For this review, take the finished solid that the model builds, in its own axes (mm). Coordinates: 2 decimals unless noted, no trailing zeros. Write each loop counter-clockwise with the first axis right and the second up, starting at its lowest first coordinate (ties: lowest second). Pieces come first, ordered by that corner, then holes. Notation, with made-up numbers: M 17,52 L 29,52 A15 ccw 29,59 Z; hole C 28.5,17.5 d3. An arc over 180 degrees is marked long. One line per question, with ' | ' between items.
from build123d import *

# Parameters (mm, degrees)
RESSALTO_EXTRUS_O1_DEPTH = 6
FILETE1_R                = 80
CORTE_EXTRUS_O1_DEPTH    = 496.818515185
FILETE2_R                = 80
CORTE_EXTRUS_O2_DEPTH    = 496.818515327
CORTE_EXTRUS_O3_DEPTH    = 6
ESBO_O7_W                = 100
ESBO_O7_H                = 10
RESSALTO_EXTRUS_O4_DEPTH = 6


with BuildPart() as part:
    # Esboço1 → Ressalto-extrusão1 (new body)
    with BuildSketch(Plane.XY):
        Polygon((-150, 70), (0, 70), (0, 0), (180, 0), (180, 70), (330, 70), (330, 370), (-150, 370), align=None)
    extrude(amount=RESSALTO_EXTRUS_O1_DEPTH)

    # Filete1
    filete1_edges = [part.edges().sort_by_distance(p)[0] for p in [
        (-150, 370, 3),
        (330, 370, 3),
    ]]
    fillet(filete1_edges, radius=FILETE1_R)

    # Esboço4 → Corte-extrusão1 (cut, through all)
    with BuildSketch(Plane.XY.offset(6)):
        with BuildLine():
            Line((-150, 70), (0, 70))
            ThreePointArc((0, 70), (-36.716416622, 160.567770202), (-126.135181443, 200))
            Line((-126.135181443, 200), (-150, 200))
            Line((-150, 200), (-150, 70))
        make_face()
        with BuildLine():
            Line((330, 200), (306.135181443, 200))
            ThreePointArc((306.135181443, 200), (216.716416622, 160.567770202), (180, 70))
            Line((180, 70), (330, 70))
            Line((330, 70), (330, 200))
        make_face()
    extrude(amount=-CORTE_EXTRUS_O1_DEPTH, mode=Mode.SUBTRACT)

    # Filete2
    filete2_edges = [part.edges().sort_by_distance(p)[0] for p in [
        (330, 200, 3),
        (-150, 200, 3),
    ]]
    fillet(filete2_edges, radius=FILETE2_R)

    # Esboço5 → Corte-extrusão2 (cut, through all)
    with BuildSketch(Plane.XY.offset(6)):
        with BuildLine():
            Line((254.973969337, 280), (-76.120192614, 280))
            ThreePointArc((-76.120192614, 280), (-81.120192614, 275), (-76.120192614, 270))
            Line((-76.120192614, 270), (254.973969337, 270))
            ThreePointArc((254.973969337, 270), (259.973969337, 275), (254.973969337, 280))
        make_face()
    extrude(amount=-CORTE_EXTRUS_O2_DEPTH, mode=Mode.SUBTRACT)

    # Esboço6 → Corte-extrusão3 (cut)
    with BuildSketch(Plane.XY.offset(6)):
        with BuildLine():
            Line((50, 70), (130, 70.020316047))
            ThreePointArc((130, 70.020316047), (144.44257782, 140.677589128), (185.453428357, 200))
            Line((185.453428357, 200), (-5.474624038, 200))
            ThreePointArc((-5.474624038, 200), (35.551661067, 140.670775275), (50, 70))
        make_face()
    extrude(amount=-CORTE_EXTRUS_O3_DEPTH, mode=Mode.SUBTRACT)

    # Esboço7 → Ressalto-extrusão4 (add)
    with BuildSketch(Plane.XY.offset(6)):
        with Locations((89.426888362, 275)):
            Rectangle(ESBO_O7_W, ESBO_O7_H)
    extrude(amount=-RESSALTO_EXTRUS_O4_DEPTH)


solid = part.part
1) To check wall thickness, follow line 1 along Y through (x, z) = (51, 5.5); line 2 along Y through (x, z) = (22.5, 5.25); line 3 along Y through (x, z) = (155.5, 3.5). State the ranges of each line that lie inside material, in increasing order. Write a range as [from, to].
Responses:
line 1: [0, 70], [200, 370] | line 2: [0, 165.64], [200, 270], [280, 370] | line 3: [0, 162.39], [200, 270], [280, 370]
2) We need section B-B on x = 116.5. State the section outline as (y, z) points, then the cut area to 3 significant figures.
Responses:
outline: M 0,0 L 70.02,0 L 70.02,6 L 0,6 Z; M 200,0 L 370,0 L 370,6 L 200,6 Z | area: 1,440 mm^2
3) We need section C-C on z = 1. State how many separate pieces and enclosed holes the cut face has, then the cut area to 3 significant figures.
Responses:
separate pieces: 1 | enclosed holes: 3 | area: 103,000 mm^2
4) We need section A-A on y = 135.5. State the section outline as (x, z) points, then the cut area to 3 significant figures.
Responses:
outline: M -17.7,0 L 37.66,0 L 37.66,6 L -17.7,6 Z; M 142.33,0 L 197.7,0 L 197.7,6 L 142.33,6 Z | area: 664 mm^2
5) We need section D-D on y = 63. State the section outline as (x, z) points, then the cut area to 3 significant figures.
Responses:
outline: M 0,0 L 180,0 L 180,6 L 0,6 Z | area: 1,080 mm^2
6) Insertion check: pin 1 Ø1 at (x, z) = (-99.5, 5.5) entering from -Y. The pin has a flat end and moves straight along its axis. Give the tip position at first contact, or say it passes through.
Responses:
pin 1: y = 196.73
7) The part is to be moulded in two halves that separate along Y. For faces 1 (the flat face through (87, 229, 0)), 2 (the cylindrical face through (-125.94, 347.19, 3.04)), 3 (the cylindrical face through (35.15, 141.6, 3.04)), say which applies: +Y half, -Y half, draft (parallel to the pull), parting line (faces both ways), or undercut.
Responses:
face 1: draft | face 2: +Y half | face 3: undercut
